Could you check a few things on this model? Use its own coordinates, in mm. A direction names the side the tool comes from. Coordinates: 2 decimals unless noted, no trailing zeros. Order: outer loops, then holes, each group sorted by start corner. A loop starts at its lowest first (then second) coordinate and runs counter-clockwise, first axis right, second up. Notation, with made-up numbers: (78.25, -30.75) - (101.25, -30.75) arc R22 ccw to (101.25, -7.75) - close; hole circle Ø3 at (-20, 50). An arc over 180 degrees is marked (long way). One line per item, written item: value.
from build123d import *

# Parameters (mm, degrees)
F0_W     = 92.31437
F0_H     = 83.259412
F1_DEPTH = 50.8
F4_DEPTH = 127
F5_DEPTH = 10.16
F7_DEPTH = 10.16
F8_R     = 7.158054
F8_R_2   = 7.413985
F9_DEPTH = 152.4


with BuildPart() as f1:
    # F0 (on Top) → F1 (new body)
    with BuildSketch(Plane.XY):
        Rectangle(F0_W, F0_H)
    extrude(amount=F1_DEPTH)

    # F2 (on face) → F4 (cut)
    with BuildSketch(Plane.XZ.offset(41.629706)):
        with BuildLine():
            Line((20.920252, 50.8), (-20.920252, 50.8))
            ThreePointArc((-20.920252, 50.8), (0, 29.879748), (20.920252, 50.8))
        make_face()
    extrude(amount=-F4_DEPTH, mode=Mode.SUBTRACT)

    # F3 (on face) → F5 (join)
    with BuildSketch(Plane.XZ.offset(41.629706)):
        with BuildLine():
            Line((-20.920252, 50.8), (-29.502509, 50.8))
            ThreePointArc((-29.502509, 50.8), (0, 21.343507), (29.502509, 50.8))
            Line((29.502509, 50.8), (20.920252, 50.8))
            ThreePointArc((20.920252, 50.8), (0, 29.879748), (-20.920252, 50.8))
        make_face()
    extrude(amount=F5_DEPTH)

    # F6 (on face) → F7 (join)
    with BuildSketch(Plane(origin=(0, 41.629706, 0), x_dir=(-1, 0, 0), z_dir=(0, 1, 0))):
        with BuildLine():
            Line((-20.920252, 50.8), (-28.88168, 50.8))
            ThreePointArc((-28.88168, 50.8), (0, 21.91832), (28.88168, 50.8))
            Line((28.88168, 50.8), (20.920252, 50.8))
            ThreePointArc((20.920252, 50.8), (0, 29.879748), (-20.920252, 50.8))
        make_face()
    extrude(amount=F7_DEPTH)

    # F8 (on face) → F9 (cut)
    with BuildSketch(Plane.XY.offset(50.8)):
        with Locations((33.635359, 0)):
            Circle(F8_R)
        with Locations((-34.185261, 0)):
            Circle(F8_R_2)
    extrude(amount=-F9_DEPTH, mode=Mode.SUBTRACT)


solid = f1.part
Item 1: I want a section at D-D on z = 14. Please give me the cut outline in (x, y), then the cut area to 3 significant figures.
Conclusion:
outline: (-46.16, -41.63) - (46.16, -41.63) - (46.16, 41.63) - (-46.16, 41.63) - close; hole circle Ø14.83 at (-34.19, 0); hole circle Ø14.32 at (33.64, 0)
area: 7,350 mm²
Item 2: If I drill on probe 1 along Y at (x, z) = (33, 38); probe 2 along X at (y, z) = (11.5, 31.5); probe 3 along Y at (x, z) = (-6, 13), over which ranges is the centre line in solid material (lowest first)?
Conclusion:
probe 1: -41.63 to -7.13, 7.13 to 41.63
probe 2: -46.16 to -8.07, 8.07 to 46.16
probe 3: -41.63 to 41.63
Item 3: Thinking about a two-plate mould opening in X: for faces 4 (the face through (-0.46, -0.725, 29.885)), 5 (the face through (-46.157, -1, 25)), 6 (the face through (40.463, 2.15, 25.756)), 7 (the face through (-0.4, -51.79, 29.7)), which applies, pulls with the +X half, pulls with the -X half, needs draft (parallel to the pull), parting line crosses it, or undercut?
Conclusion:
face 4: undercut
face 5: pulls with the -X half
face 6: undercut
face 7: needs draft
Item 4: For faces 1 (the face through (-0.65, -46.64, 21.35)), 2 (the face through (0.635, 46.639, 21.925)), 3 (the face through (46.157, -1, 25)), which set-ups out of +Z, -Z, +X, -X, +Y, -Y let a thin tool reach every point of the face, with its end or its side?
Conclusion:
face 1: -Z, -Y
face 2: -Z, +Y
face 3: +Z, -Z, +X, +Y, -Y
Item 5: I want a section at B-B on x = 37.5. Please give me the cut outline in (y, z).
Conclusion:
outline: (-41.63, 0) - (-6.03, 0) - (-6.03, 50.8) - (-41.63, 50.8) - close; (6.03, 0) - (41.63, 0) - (41.63, 50.8) - (6.03, 50.8) - close
Item 6: I want a section at A-A on y = 0. Please give me the cut outline in (x, z).
Conclusion:
outline: (-46.16, 0) - (-41.6, 0) - (-41.6, 50.8) - (-46.16, 50.8) - close; (-26.77, 0) - (26.48, 0) - (26.48, 50.8) - (20.92, 50.8) arc R20.92 cw to (-20.92, 50.8) - (-26.77, 50.8) - close; (40.79, 0) - (46.16, 0) - (46.16, 50.8) - (40.79, 50.8) - close
Item 7: I want a section at C-C on z = 36. Please give me the cut outline in (x, y) (3 decimals).
Conclusion:
outline: (-46.157, -41.63) - (-25.495, -41.63) - (-25.495, -51.79) - (-14.786, -51.79) - (-14.786, 51.79) - (-24.801, 51.79) - (-24.801, 41.63) - (-46.157, 41.63) - close; (14.786, -51.79) - (25.495, -51.79) - (25.495, -41.63) - (46.157, -41.63) - (46.157, 41.63) - (24.801, 41.63) - (24.801, 51.79) - (14.786, 51.79) - close; hole circle Ø14.828 at (-34.185, 0); hole circle Ø14.316 at (33.635, 0)
Item 8: I'm going to push a flat-ended pin straight in: pin 1 Ø1 at (x, z) = (1, 8) entering from +Y. Where does the tip first touch, or does it pass through?
Conclusion:
pin 1: y = 41.63
